Geometry check sheet. Reference: the model listing, model coordinates, mm. Face numbers are marked on the shaded views. A direction names the side the tool comes from. Give positions to 0.01 mm unless a question says otherwise; leave off trailing zeros. Write each loop counter-clockwise with the first axis right and the second up, starting at its lowest first coordinate (ties: lowest second). Pieces come first, ordered by that corner, then holes. Notation, with made-up numbers: M 3.5,-24 L 10.5,-24 A6 ccw 10.5,-16 Z; hole C 40,88.5 d8. An arc over 180 degrees is marked long. One line per item, written item: value. Start each with the question number.
1. Tool access check on the marked faces 1, 2 and 3. Record the directions out of +Z, -Z, +X, -X, +Y, -Y that give a thin tool (end or side, any length) a straight path to the whole face; none if there is none.
2. Cross-section at C-C on y = 4. Record the cut outline in (x, z).
3. Release check for a two-part mould opening along Y. For the marked faces 4, 5, 6 and 7 record: pulls with the +Y half, pulls with the -Y half, needs draft (parallel to the pull), parting line crosses it, or undercut.
4. Cross-section at A-A on y = 15. Record the cut outline in (x, z).
5. Scan lines: line 1 (X direction, y = -10, z = 14.5); line 2 (Y direction, x = -37.25, z = 20); line 3 (Z direction, x = 42.5, y = 15). Record each from-to range of solid material in increasing order.
6. Cross-section at D-D on z = 5. Record the cut outline in (x, y).
7. Gauge pin test, flat ends, axial feed: pin 1 (15 mm diameter, centred on x = 11, z = 20, fed in from +Y); pin 2 (11 mm diameter, centred on y = 15, z = 20, fed in from -X). Record the tip position at first contact, or that the pin passes through.
8. Cross-section at B-B on z = 20. Record the cut outline in (x, y), then the cut area to 3 significant figures.
from build123d import *

# Parameters (mm, degrees)
F1_DEPTH      = 30
F2_R          = 6
F3_DEPTH      = 10
F3_DEPTH_BACK = 80
F4_R          = 8
F5_R          = 1


with BuildPart() as f1:
    # F0 (on Top) → F1 (new body)
    with BuildSketch(Plane.XY):
        Polygon((-14.1, -30), (-45, -30), (-45, -40.1), (-10.4239006339, -40.1), align=None)
        Polygon((45, -30), (14.1, -30), (10.4239006339, -40.1), (45, -40.1), align=None)
        Polygon((-35, 30), (-45, 30), (-45, -30), (-14.1, -30), (14.1, -30), (45, -30), (45, 30), (35, 30), (35, -20), (-35, -20), align=None)
    extrude(amount=F1_DEPTH)

    # F2 (on face) → F3 (cut, two sides)
    with BuildSketch(Plane(origin=(35, 0, 0), x_dir=(0, -1, 0), z_dir=(-1, 0, 0))) as f3_sk:
        with Locations((-15, 20)):
            Circle(F2_R)
    extrude(amount=-F3_DEPTH, mode=Mode.SUBTRACT)
    extrude(f3_sk.sketch, amount=F3_DEPTH_BACK, mode=Mode.SUBTRACT)

    # F4
    f4_edges = [f1.edges().sort_by_distance(p)[0] for p in [
        (40, 30, 30),
        (40, 30, 0),
        (-40, 30, 30),
        (-40, 30, 0),
    ]]
    fillet(f4_edges, radius=F4_R)

    # F5
    f5_edges = [f1.edges().sort_by_distance(p)[0] for p in [
        (-10.423901, -40.1, 15),
        (10.423901, -40.1, 15),
        (45, -40.1, 15),
        (-45, -40.1, 15),
    ]]
    fillet(f5_edges, radius=F5_R)


solid = f1.part
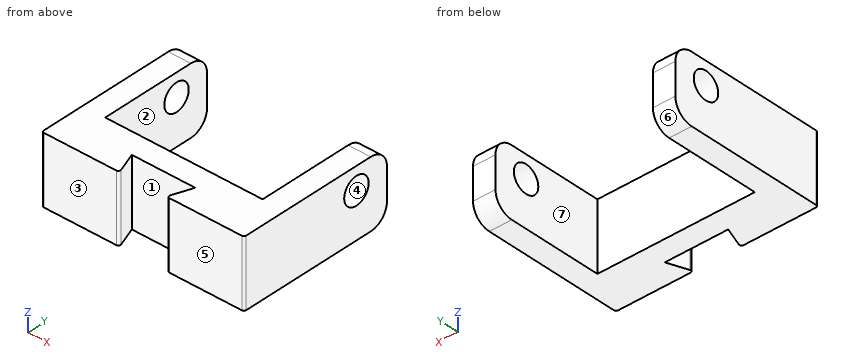
Report:
1. face 1: +Z, -Z
1. face 2: +Z, -Z, +Y
1. face 3: +Z, -Z, +X, -X, -Y
2. outline: M -45,0 L -35,0 L -35,30 L -45,30 Z; M 35,0 L 45,0 L 45,30 L 35,30 Z
3. face 4: undercut
3. face 5: pulls with the -Y half
3. face 6: pulls with the +Y half
3. face 7: needs draft
4. outline: M -45,0 L -35,0 L -35,14 L -45,14 Z; M -45,26 L -35,26 L -35,30 L -45,30 Z; M 35,0 L 45,0 L 45,14 L 35,14 Z; M 35,26 L 45,26 L 45,30 L 35,30 Z
5. line 1: x = -45 to -35, 35 to 45
5. line 2: y = -40.1 to 9, 21 to 30
5. line 3: z = 0 to 14, 26 to 30
6. outline: M -45,-39.1 A1 ccw -44,-40.1 L -11.85,-40.1 A1 ccw -10.91,-38.76 L -14.1,-30 L 14.1,-30 L 10.91,-38.76 A1 ccw 11.85,-40.1 L 44,-40.1 A1 ccw 45,-39.1 L 45,29.42 L 35,29.42 L 35,-20 L -35,-20 L -35,29.42 L -45,29.42 Z
7. pin 1: stops at y = -20
7. pin 2: passes through
8. outline: M -45,-39.1 A1 ccw -44,-40.1 L -11.85,-40.1 A1 ccw -10.91,-38.76 L -14.1,-30 L 14.1,-30 L 10.91,-38.76 A1 ccw 11.85,-40.1 L 44,-40.1 A1 ccw 45,-39.1 L 45,9 L 35,9 L 35,-20 L -35,-20 L -35,9 L -45,9 Z; M -45,21 L -35,21 L -35,30 L -45,30 Z; M 35,21 L 45,21 L 45,30 L 35,30 Z
8. area: 2,320 mm^2
